Input: part model. Units: mm. Frame: model coordinates. A direction names the side the tool comes from. Coordinates: 2 decimals unless noted, no trailing zeros. Order: outer loops, then holes, each group sorted by start corner. A loop starts at its lowest first (then second) coordinate and runs counter-clockwise, first axis right, second up. Notation, with made-up numbers: (52, 63) -> (84, 63) arc R18 ccw to (84, 95) -> close; hole circle Ø3 at (-17.5, -12). An arc over 180 degrees is marked (long way). One line per question, with ' | ' between items.
```python
from build123d import *

# Parameters (mm, degrees)
F0_W     = 10.5
F0_H     = 2.5
F0_W_2   = 8
F0_H_2   = 3.25
F1_DEPTH = 17
F2_R     = 1.6
F3_DEPTH = 25
F4_R     = 2
F5_W     = 10.5
F5_H     = 2.5
F6_DEPTH = 2


with BuildPart() as f1:
    # F0 (on Top) → F1 (new body)
    with BuildSketch(Plane.XY):
        Polygon((7, 5), (-7, 5), (-7, -1.25), (-7, -4.5), (7, -4.5), (7, -1.25), align=None)
        with Locations((0, -1.25)):
            Rectangle(F0_W, F0_H, mode=Mode.SUBTRACT)
        with Locations((11, -2.875)):
            Rectangle(F0_W_2, F0_H_2)
        with Locations((-11, -2.875)):
            Rectangle(F0_W_2, F0_H_2)
    extrude(amount=F1_DEPTH)

    # F2 (on face) → F3 (cut)
    with BuildSketch(Plane.XZ.offset(4.5)):
        with Locations((11.5, 8.5)):
            Circle(F2_R)
        with Locations((-11.5, 8.5)):
            Circle(F2_R)
    extrude(amount=-F3_DEPTH, mode=Mode.SUBTRACT)

    # F4
    f4_edges = [f1.edges().sort_by_distance(p)[0] for p in [
        (0, 5, 0),
        (-7, 5, 8.5),
        (0, 5, 17),
        (7, 5, 8.5),
        (-15, -2.875, 0),
        (15, -2.875, 0),
    ]]
    fillet(f4_edges, radius=F4_R)

    # F5 (on face) → F6 (join)
    with BuildSketch(Plane.XY.offset(17)):
        Polygon((-7, -1.25), (-15, -1.25), (-15, -4.5), (15, -4.5), (15, -1.25), (7, -1.25), (7, 3), (-7, 3), align=None)
        with Locations((0, -1.25)):
            Rectangle(F5_W, F5_H, mode=Mode.SUBTRACT)
        with Locations((0, -1.25)):
            Rectangle(F5_W, F5_H)
    extrude(amount=F6_DEPTH)


solid = f1.part
```
1. Ray query, line 1 (Z direction, x = -11.5, y = -2.2); line 2 (X direction, y = -1.5, z = 10.25); line 3 (Y direction, x = -4.25, z = 9.5). Return the intervals inside material, ascending. Write a range as [from, to].
Recorded:
line 1: z = [0, 6.9], [10.1, 19] | line 2: x = [-15, -5.25], [5.25, 15] | line 3: y = [-4.5, -2.5], [0, 5]
2. Pin query (flat end, axial travel): pin 1 Ø1.3 at (y, z) = (1, 8.5) entering from -X; pin 2 Ø1.5 at (x, y) = (2, 3.5) entering from +Z; pin 3 Ø6.5 at (x, z) = (12.5, 11.5) entering from +Y; pin 4 Ø2 at (y, z) = (0.5, 14) entering from +X. Return the tip coordinate at first contact, or that it passes through.
Recorded:
pin 1: stops at x = -7 | pin 2: stops at z = 19 | pin 3: stops at y = -1.25 | pin 4: stops at x = 7
3. Mould query, pull axis Y, two halves, no side actions, for faces 4 (the face through (0, -4.5, 9)), 5 (the face through (0, -1, 17)), 6 (the face through (0, 3, 18)). Classes: released by +Y, released by -Y, zero draft, split by the parting line, or undercut.
Recorded:
face 4: released by -Y | face 5: undercut | face 6: released by +Y
4. Access query for faces 1 (the face through (-9, -1.25, 9)), 2 (the face through (6.4, 4.43, 8.62)), 3 (the face through (-5.25, -1, 8)). Directions: +Z, -Z, +X, -X, +Y, -Y. A direction counts if a zero-diameter tool reaches every point of the face in a straight line with its end or side. Return the directions, or none.
Recorded:
face 1: +Z, -Z, -X, +Y | face 2: +Z, -Z, +X, +Y | face 3: -Z
5. Cut plane D-D, the plane z = 13. Return loops of the section in (x, y).
Recorded:
outline: (-15, -4.5) -> (15, -4.5) -> (15, -1.25) -> (7, -1.25) -> (7, 3) arc R2 ccw to (5, 5) -> (-5, 5) arc R2 ccw to (-7, 3) -> (-7, -1.25) -> (-15, -1.25) -> close; hole (-5.25, -2.5) -> (5.25, -2.5) -> (5.25, 0) -> (-5.25, 0) -> close
6. Cut plane A-A, the plane x = 11.5. Return loops of the section in (y, z), and give its area (4 significant figures).
Recorded:
outline: (-4.5, 0) -> (-1.25, 0) -> (-1.25, 6.9) -> (-4.5, 6.9) -> close; (-4.5, 10.1) -> (-1.25, 10.1) -> (-1.25, 19) -> (-4.5, 19) -> close | area: 51.35 mm^2
7. Cut plane C-C, the plane y = -1.75. Return loops of the section in (x, z), and give its area (3 significant figures).
Recorded:
outline: (-15, 2) arc R2 ccw to (-13, 0) -> (-5.25, 0) -> (-5.25, 17) -> (5.25, 17) -> (5.25, 0) -> (13, 0) arc R2 ccw to (15, 2) -> (15, 19) -> (-15, 19) -> close; hole circle Ø3.2 at (-11.5, 8.5); hole circle Ø3.2 at (11.5, 8.5) | area: 374 mm^2
8. Cut plane B-B, the plane z = 8.5. Return loops of the section in (x, y), and give its area (3 significant figures).
Recorded:
outline: (-15, -4.5) -> (-13.1, -4.5) -> (-13.1, -1.25) -> (-15, -1.25) -> close; (-9.9, -4.5) -> (9.9, -4.5) -> (9.9, -1.25) -> (7, -1.25) -> (7, 3) arc R2 ccw to (5, 5) -> (-5, 5) arc R2 ccw to (-7, 3) -> (-7, -1.25) -> (-9.9, -1.25) -> close; (13.1, -4.5) -> (15, -4.5) -> (15, -1.25) -> (13.1, -1.25) -> close; hole (-5.25, -2.5) -> (5.25, -2.5) -> (5.25, 0) -> (-5.25, 0) -> close | area: 136 mm^2
